Geometry: final body of the model. Coordinates: model frame, mm. A direction names the side the tool comes from. Give positions to 0.01 mm unless a question says otherwise; leave off trailing zeros. Order: outer loops, then holes, each group sorted by start corner. A loop starts at its lowest first (then second) coordinate and runs counter-clockwise, first axis right, second up. Notation, with made-up numbers: (25, -39.5) -> (81, -39.5) arc R9 ccw to (81, -33.5) -> close; hole circle Ø1 at (23.25, 81.25). An arc over 180 degrees is marked (long way). Answer in a Markdown table with one row per item. Add a question column.
Q1. Contact query for flat-ended pins moving along their axis: P1, Ø12, axis at y = 7, z = 28.5, coming from the -X side; P2, Ø0.9, axis at x = -3.5, z = 35, coming from the +Y side; P3, Ø0.7, axis at y = 16, z = 19, coming from the +X side. Output: stop coordinate, or through.
Q2. Cut plane A-A on y = 0. Return the cut outline in (x, z).
Q3. Pull-direction query (Y, two-part tool) for faces 1 (the face through (-11.59, -11.31, 24.65)), 2 (the face through (-0.3, -27.5, 22.2)), 3 (the face through (18.69, -9.06, 24.65)), 4 (the face through (4, 24.12, 24)); classes: +Y half, -Y half, draft (parallel to the pull), parting line (faces both ways), or undercut.
Q4. Cut plane B-B on x = 0. Return the cut outline in (y, z), and give its area (3 significant figures).
Q5. Line query: line 1 along Y through (x, z) = (0, 37.5); line 2 along Y through (x, z) = (7, 48); line 3 along X through (y, z) = (-19, 5). Output: solid intervals per line, ascending. Write a range as from..to.
Q6. Set-up query: faces 5 (the face through (-19.055, -15.237, 23.803)), 6 (the face through (-22.723, -8.883, 23.803)), 7 (the face through (-1.5, 21, 25)), 8 (the face through (0, 14.12, 25)), 9 (the face through (19.55, -17.64, 23.36)). Return all of +Z, -Z, +X, -X, +Y, -Y with unobstructed straight access to the full face (end or side cutting, diameter ignored); none if empty.
from build123d import *

# Parameters (mm, degrees)
SKETCH_R     = 27.5
SKETCH_R_2   = 10
PAD_DEPTH    = 50
CHAMFER_SIZE = 5
POCKET_DEPTH = 50.001


with BuildPart() as part:
    # Sketch → Pad (new body)
    with BuildSketch(Plane.XY):
        Circle(SKETCH_R)
        Circle(SKETCH_R_2, mode=Mode.SUBTRACT)
    extrude(amount=PAD_DEPTH)

    # Chamfer
    chamfer_edges = [part.edges().sort_by_distance(p)[0] for p in [
        (-27.5, 0, 50),
    ]]
    chamfer(chamfer_edges, length=CHAMFER_SIZE)

    # Sketch001 → Pocket (cut, through all)
    with BuildSketch(Plane(origin=(0, 0, 0), x_dir=(1, 0, 0), z_dir=(0, 0, -1))):
        with BuildLine():
            Line((5.5, -27.883587), (5.5, -24.511159))
            ThreePointArc((5.5, -24.511159), (5.385432, -24.234568), (5.108841, -24.12))
            Line((5.108841, -24.12), (2.186238, -24.12))
            ThreePointArc((1.5, -23.433762), (1.700994, -23.919006), (2.186238, -24.12))
            Line((1.5, -23.433762), (1.5, -17.926959))
            Line((1.5, -17.926959), (2.294017, -17.926959))
            Line((2.294017, -17.926959), (2.294017, -17.12))
            Line((2.294017, -17.12), (3.752143, -17.12))
            ThreePointArc((3.752143, -17.12), (3.927404, -17.047404), (4, -16.872143))
            Line((4, -16.872143), (4, -14.488966))
            ThreePointArc((4, -14.488966), (3.891932, -14.228068), (3.631034, -14.12))
            Line((3.631034, -14.12), (-3.631034, -14.12))
            ThreePointArc((-3.631034, -14.12), (-3.891932, -14.228068), (-4, -14.488966))
            Line((-4, -16.872143), (-4, -14.488966))
            ThreePointArc((-4, -16.872143), (-3.927404, -17.047404), (-3.752143, -17.12))
            Line((-3.752143, -17.12), (-2.294017, -17.12))
            Line((-2.294017, -17.926959), (-2.294017, -17.12))
            Line((-2.294017, -17.926959), (-1.5, -17.926959))
            Line((-1.5, -23.433762), (-1.5, -17.926959))
            ThreePointArc((-2.186238, -24.12), (-1.700994, -23.919006), (-1.5, -23.433762))
            Line((-5.108841, -24.12), (-2.186238, -24.12))
            ThreePointArc((-5.108841, -24.12), (-5.385432, -24.234568), (-5.5, -24.511159))
            Line((-5.5, -27.883587), (-5.5, -24.511159))
            Line((-5.5, -27.883587), (5.5, -27.883587))
        make_face()
        with BuildLine():
            Line((21.397895, 18.704933), (18.477287, 17.018719))
            ThreePointArc((18.477287, 17.018719), (18.295036, 16.781205), (18.334112, 16.484386))
            Line((18.334112, 16.484386), (19.795414, 13.953338))
            ThreePointArc((19.544233, 13.01592), (19.863969, 13.432608), (19.795414, 13.953338))
            Line((19.544233, 13.01592), (14.775202, 10.262518))
            Line((14.775202, 10.262518), (14.378193, 10.950156))
            Line((14.378193, 10.950156), (13.679346, 10.546677))
            Line((13.679346, 10.546677), (12.950283, 11.809451))
            ThreePointArc((12.950283, 11.809451), (12.799783, 11.924934), (12.611704, 11.900173))
            Line((12.611704, 11.900173), (10.547813, 10.708585))
            ThreePointArc((10.547813, 10.708585), (10.375902, 10.484546), (10.412762, 10.204568))
            Line((10.412762, 10.204568), (14.043796, 3.915432))
            ThreePointArc((14.043796, 3.915432), (14.267834, 3.743521), (14.547813, 3.780381))
            Line((16.611705, 4.971969), (14.547813, 3.780381))
            ThreePointArc((16.611705, 4.971969), (16.727187, 5.12247), (16.702426, 5.310548))
            Line((16.702426, 5.310548), (15.973363, 6.573323))
            Line((16.67221, 6.976803), (15.973363, 6.573323))
            Line((16.67221, 6.976803), (16.275202, 7.664442))
            Line((21.044233, 10.417843), (16.275202, 7.664442))
            ThreePointArc((21.981652, 10.166663), (21.564963, 10.486398), (21.044233, 10.417843))
            Line((23.442954, 7.635614), (21.981652, 10.166663))
            ThreePointArc((23.442954, 7.635614), (23.680468, 7.453363), (23.977287, 7.492439))
            Line((26.897895, 9.178654), (23.977287, 7.492439))
            Line((26.897895, 9.178654), (21.397895, 18.704933))
        make_face()
        with BuildLine():
            Line((-26.897895, 9.178654), (-23.977287, 7.492439))
            ThreePointArc((-23.977287, 7.492439), (-23.680468, 7.453363), (-23.442954, 7.635614))
            Line((-23.442954, 7.635614), (-21.981652, 10.166662))
            ThreePointArc((-21.044233, 10.417843), (-21.564964, 10.486398), (-21.981652, 10.166662))
            Line((-21.044233, 10.417843), (-16.275202, 7.664441))
            Line((-16.275202, 7.664441), (-16.67221, 6.976803))
            Line((-16.67221, 6.976803), (-15.973363, 6.573323))
            Line((-15.973363, 6.573323), (-16.702426, 5.310548))
            ThreePointArc((-16.702426, 5.310548), (-16.727188, 5.12247), (-16.611705, 4.971969))
            Line((-16.611705, 4.971969), (-14.547813, 3.780381))
            ThreePointArc((-14.547813, 3.780381), (-14.267835, 3.743521), (-14.043796, 3.915432))
            Line((-14.043796, 3.915432), (-10.412762, 10.204568))
            ThreePointArc((-10.412762, 10.204568), (-10.375902, 10.484547), (-10.547813, 10.708585))
            Line((-12.611705, 11.900174), (-10.547813, 10.708585))
            ThreePointArc((-12.611705, 11.900174), (-12.799783, 11.924935), (-12.950284, 11.809451))
            Line((-12.950284, 11.809451), (-13.679346, 10.546677))
            Line((-14.378193, 10.950156), (-13.679346, 10.546677))
            Line((-14.378193, 10.950156), (-14.775202, 10.262518))
            Line((-19.544233, 13.015919), (-14.775202, 10.262518))
            ThreePointArc((-19.795414, 13.953338), (-19.863969, 13.432608), (-19.544233, 13.015919))
            Line((-18.334112, 16.484386), (-19.795414, 13.953338))
            ThreePointArc((-18.334112, 16.484386), (-18.295036, 16.781205), (-18.477287, 17.018719))
            Line((-21.397895, 18.704933), (-18.477287, 17.018719))
            Line((-21.397895, 18.704933), (-26.897895, 9.178654))
        make_face()
    extrude(amount=-POCKET_DEPTH, mode=Mode.SUBTRACT)


solid = part.part
Completed:
| question | item | result |
|---|---|---|
| 1 | P1 | stops at x = -27.48 |
| 1 | P2 | stops at y = 24.12 |
| 1 | P3 | stops at x = 22.61 |
| 2 | outline | (-27.5, 0) -> (-10, 0) -> (-10, 50) -> (-22.5, 50) -> (-27.5, 45) -> close; (10, 0) -> (27.5, 0) -> (27.5, 45) -> (22.5, 50) -> (10, 50) -> close |
| 3 | face 1 | undercut |
| 3 | face 2 | -Y half |
| 3 | face 3 | undercut |
| 3 | face 4 | +Y half |
| 4 | outline | (-27.5, 0) -> (-10, 0) -> (-10, 50) -> (-22.5, 50) -> (-27.5, 45) -> close; (10, 0) -> (14.12, 0) -> (14.12, 50) -> (10, 50) -> close |
| 4 | area | 1,070 mm² |
| 5 | line 1 | y = -27.5..-10, 10..14.12 |
| 5 | line 2 | y = -23.48..-7.14, 7.14..23.48 |
| 5 | line 3 | x = -19.88..19.88 |
| 6 | face 5 | +Z, -Z, -X |
| 6 | face 6 | +Z, -Z, -Y |
| 6 | face 7 | +Z, -Z, +Y |
| 6 | face 8 | +Z, -Z |
| 6 | face 9 | +Z, -Z, +X |
